Verification items for the finished model (mm, model axes). A direction names the side the tool comes from. Give positions to 0.01 mm unless a question says otherwise; leave off trailing zeros. Loops run counter-clockwise (first coordinate to the right, second up) from the corner with the lowest first, then second, coordinate; pieces in that order, holes last. Notation, with made-up numbers: M -29.5,-4.5 L 4.5,-4.5 A13 ccw 4.5,4.5 Z; hole C 36.25,-30 d4. An arc over 180 degrees is marked long. Use CSV: the item, a comma, the result in double quotes.
from build123d import *

# Parameters (mm, degrees)
F2_R = 5.08
F3_R = 5.08


# Not quite as in the source:
# - a fillet or chamfer that OpenCascade refuses, or shapes differently, is made with other operations: its cross-section is extruded or revolved along the edge and cut away or added


with BuildPart() as f1:
    # F0 (on Front) → F1 (revolve)
    with BuildSketch(Plane.XZ):
        Polygon((68.2647973299, 48.6955605447), (59.4662241638, 48.6955605447), (59.4662241638, -48.6955568194), (0, -60.2247230709), (0, -68.4164986014), (68.2647973299, -53.5499453545), align=None)
    revolve(axis=Axis((0, 0, 0.9102020413), (0, 0, -1)))

    # F2
    f2_edges = [f1.edges().sort_by_distance(p)[0] for p in [
        (-59.466224, 0, -48.695557),
        (29.733112, 0, -54.46014),
    ]]
    fillet(f2_edges, radius=F2_R)

    # F3
    f3_edges = [f1.edges().sort_by_distance(p)[0] for p in [
        (-59.466224, 0, 48.695561),
    ]]
    fillet(f3_edges, radius=F3_R)

    # F4: fillet of radius 5.08 on 1 edges, made by hand

    # F4_s1 → F4_t2 (revolve, cut)
    with BuildSketch(Plane.XZ):
        with BuildLine():
            ThreePointArc((64.5462241638, 48.6955605447), (67.2296983371, 46.8746892895), (68.2647973299, 43.8013888093))
            Line((68.2647973299, 43.8013888093), (68.2647973299, 48.6955605447))
            Line((68.2647973299, 48.6955605447), (64.5462241638, 48.6955605447))
        make_face()
    revolve(axis=Axis((0, 0, 48.6955605447), (0, 0, -1)), mode=Mode.SUBTRACT)


solid = f1.part
(1) Scan lines: L1, parallel to X at y = 0, z = -9; L2, parallel to X at y = 52, z = 14.5. Record each from-to range of solid material in increasing order. Write a range as from..to.
Calculated:
L1,"x = -68.26..-59.47, 59.47..68.26"
L2,"x = -44.23..-28.85, 28.85..44.23"
(2) Section check A-A on z = 28. Record the cut outline in (x, y).
Calculated:
outline,"C 0,0 d136.53; hole C 0,0 d118.93"
(3) Tool access check on faces 3 (the cylindrical face through (65.112, -20.505, -4.193)), 4 (the cylindrical face through (27.44, 52.757, -1.062)). Record the directions out of +Z, -Z, +X, -X, +Y, -Y that give a thin tool (end or side, any length) a straight path to the whole face; none if there is none.
Calculated:
face 3,"+Z, -Z"
face 4,"+Z"
(4) Section check B-B on z = -56.5. Record the cut outline in (x, y).
Calculated:
outline,"C 0,0 d109.44; hole C 0,0 d38.42"
(5) Mould release check, pull along X, two halves, no side actions. Record for faces 1 (the conical face through (2.564, -0.807, -59.704)), 2 (the conical face through (1.971, 3.789, -67.487)): released by +X, released by -X, zero draft, split by the parting line, or undercut.
Calculated:
face 1,"undercut"
face 2,"split by the parting line"
(6) Depth check by flat-ended pin: pin 1 Ø2 at (x, z) = (-22.5, 21.5) entering from -Y; pin 2 Ø2 at (x, y) = (-43.5, 31) entering from -Z; pin 3 Ø4 at (x, y) = (47.5, -51) entering from +Z; pin 4 Ø8 at (y, z) = (3.5, -19.5) entering from -X. Enter the tip coordinate at first touch or a pass-through.
Calculated:
pin 1,"stops at y = -64.79"
pin 2,"stops at z = -57"
pin 3,"stops at z = 46.14"
pin 4,"stops at x = -68.26"
